Part model, mm, in its own coordinate system. Round coordinates to 2 decimals unless told otherwise and drop trailing zeros. Order: outer loops, then holes, each group sorted by start corner. A loop starts at its lowest first (then second) coordinate and runs counter-clockwise, first axis right, second up. Notation, with made-up numbers: (-26.75, 28.5) -> (-21.75, 28.5) arc R23 ccw to (-21.75, 58.5) -> close; hole circle Ø7 at (62.25, 25.25). An arc over 180 degrees is marked (long way). Answer as a JSON object with one key per item and string values. Group by question number.
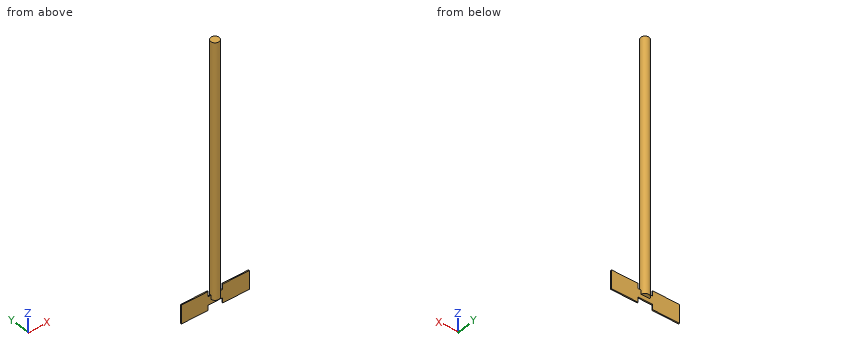
```python
from build123d import *

# Parameters (mm, degrees)
F0_W     = 85.7623966645
F0_H     = 50.8
F2_DEPTH = 3.175
F1_R     = 25.4
F4_DEPTH = 1549.4


# Not quite as in the source:
# - the program builds the solid bodies; features that only make, move or delete a surface that nothing else refers to are left out


with BuildPart() as f2:
    # F0 (on Front) → F2 (new body, symmetric)
    with BuildSketch(Plane.XZ):
        Rectangle(F0_W, F0_H)
        Polygon((42.8811983322, 56.6644097805), (42.8811983322, 25.4), (42.8811983322, -25.4), (42.8811983322, -56.6644097805), (203.2, -56.6644097805), (203.2, 56.6644097805), align=None)
        Polygon((-42.8811983322, -25.4), (-42.8811983322, 25.4), (-42.8811983322, 56.6644097805), (-203.2, 56.6644097805), (-203.2, -56.6644097805), (-42.8811983322, -56.6644097805), align=None)
    extrude(amount=F2_DEPTH, both=True)

    # F1 (on Top) → F4 (join)
    with BuildSketch(Plane.XY):
        Circle(F1_R)
    extrude(amount=F4_DEPTH)


solid = f2.part
```
Q1. Band-saw the part on B-B (y = -15). List the corners of the cut face in (x, z).
Q2. Band-saw the part on A-A (x = 0). List the corners of the cut face in (y, z) (3 decimals), plus the area to 3 significant figures.
Q3. Band-saw the part on D-D (x = -139.5). List the corners of the cut face in (y, z) (3 decimals), plus the area to 3 significant figures.
Q4. Wall check: line 1 (X direction, y = 1.5, z = 766); line 2 (X direction, y = -2.5, z = 359.5); line 3 (Z direction, x = 145, y = 1). Give the ranges that are in metal, low to high. Write a range as [from, to].
Q5. Drop flat-ended pins along their axis: pin 1 Ø5 at (x, y) = (-107.5, 0) entering from +Z; pin 2 Ø2 at (y, z) = (19, 733) entering from +X; pin 3 Ø1.9 at (x, y) = (-16, 1) entering from -Z. Give the stop position or say it passes through.
Q6. Band-saw the part on C-C (z = 1186.5). List the corners of the cut face in (x, y).
Completed:
{
 "1": {"outline": "(-20.5, 0) -> (20.5, 0) -> (20.5, 1549.4) -> (-20.5, 1549.4) -> close"},
 "2": {"outline": "(-25.4, 0) -> (-3.175, 0) -> (-3.175, -25.4) -> (3.175, -25.4) -> (3.175, 0) -> (25.4, 0) -> (25.4, 1549.4) -> (-25.4, 1549.4) -> close", "area": "78,900 mm2"},
 "3": {"outline": "(-3.175, -56.664) -> (3.175, -56.664) -> (3.175, 56.664) -> (-3.175, 56.664) -> close", "area": "720 mm2"},
 "4": {"line 1": "[-25.36, 25.36]", "line 2": "[-25.28, 25.28]", "line 3": "[-56.66, 56.66]"},
 "5": {"pin 1": "z = 56.66", "pin 2": "x = 17.92", "pin 3": "z = -25.4"},
 "6": {"outline": "circle Ø50.8 at (0, 0)"}
}
